Build history of the part. All positions in model axes, mm. Face numbers are marked on the shaded views. A direction names the side the tool comes from. Coordinates: 2 decimals unless noted, no trailing zeros. Loops run counter-clockwise (first coordinate to the right, second up) from the corner with the lowest first, then second, coordinate; pieces in that order, holes last.
Item 1: Mould opens along X. For the marked faces 4, 5 and 6 say: released by +X, released by -X, zero draft, split by the parting line, or undercut.
Item 2: Cut at D-D (x = 26). List the corners of the cut face in (y, z).
Item 3: Cut at A-A (x = 0). List the corners of the cut face in (y, z).
Item 4: Cut at B-B (z = -21). List the corners of the cut face in (x, y).
Item 5: 3-axis set-ups, long thin cutter, end or side, ignore diameter. For the marked faces 1, 2 and 3: which of +Z, -Z, +X, -X, +Y, -Y reach the whole face in a straight line?
Item 6: Flat gauge pins, fed straight in: pin 1 (3 mm diameter, centred on x = 30, y = -15, fed in from +Z); pin 2 (6.5 mm diameter, centred on x = 0, z = -21, fed in from +Y); pin 3 (24 mm diameter, centred on x = -20, y = -10.5, fed in from -Z); pin 4 (3 mm diameter, centred on x = 0, z = -21, fed in from -Y). Where does each tip first touch, or does it go through?
Item 7: Cut at C-C (y = 0). List the corners of the cut face in (x, z).
Item 8: Drill centre lines: line 1 along Z through (x, y) = (0, 3.05); line 2 along Y through (x, z) = (0, -24); line 3 along Z through (x, y) = (-27, 26). Where is each one in solid material? Low to high.
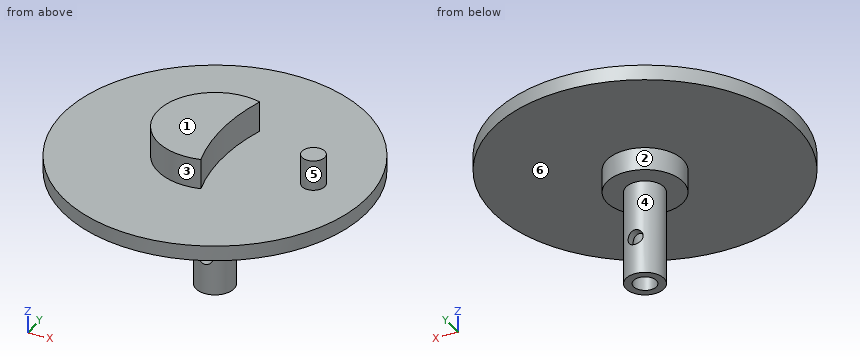
Autodesk Inventor part; units mm, degrees
ref_plane "YZ Plane" through (0, 0, 0) normal (1, 0, 0) x (0, 1, 0)
ref_plane "XZ Plane" through (0, 0, 0) normal (0, 1, 0) x (-1, 0, 0)
ref_plane "XY Plane" through (0, 0, 0) normal (0, 0, 1) x (1, 0, 0)
sketch "Sketch1" plane through (0, 0, 0) normal (0, 0, 1) x (1, 0, 0)
  circle A0 centre (0, 0) radius 40
  dimension "d0" = 40
extrude "Extrusion1" add sketch "Sketch1" along normal blind 4
sketch "Sketch2" plane through (0, 0, 4) normal (0, 0, 1) x (1, 0, 0)
  arc A0 (4.0325, 14.4478) -> (4.0325, -14.4478) centre (0, 0) ccw
  arc A1 (4.0325, 14.4478) -> (4.0325, -14.4478) centre (54.3652, 0) ccw
  dimension "d3" = 15
extrude "Extrusion2" add sketch "Sketch2" along normal blind 8
sketch "Sketch3" plane through (0, 0, 4) normal (0, 0, 1) x (1, 0, 0)
  circle A0 centre (26, 0) radius 3
  point P0 (0, 0)
  dimension "d6" = 3
sketch "Sketch4" plane through (0, 0, 0) normal (0, 0, -1) x (-1, 0, 0)
  circle A0 centre (0, 0) radius 10
  dimension "d9" = 10
extrude "Extrusion4" add sketch "Sketch4" along normal blind 6
sketch "Sketch5" plane through (0, 0, -6) normal (0, 0, -1) x (-1, 0, 0)
  circle A0 centre (0, 0) radius 5
  circle A1 centre (0, 0) radius 3
  dimension "d12" = 5
  dimension "d13" = 3
extrude "Extrusion5" add sketch "Sketch5" along normal blind 25
sketch "Sketch6" plane through (0, 0, 0) normal (0, 1, 0) x (-1, 0, 0)
  circle A0 centre (0, -21) radius 2
  point P0 (0, 0)
  dimension "d16" = 2
extrude "Extrusion6" cut sketch "Sketch6" along normal mid plane 25
extrude "Extrusion7" add sketch "Sketch3" along normal blind 8
properties part number "driverwheel"
Filled sheet:
1. face 4: split by the parting line
1. face 5: undercut
1. face 6: zero draft
2. outline: (-30.4, 0) - (30.4, 0) - (30.4, 4) - (3, 4) - (3, 12) - (-3, 12) - (-3, 4) - (-30.4, 4) - close
3. outline: (-40, 0) - (-10, 0) - (-10, -6) - (-5, -6) - (-5, -19) - (-3, -19) - (-3, -6) - (3, -6) - (3, -19) - (5, -19) - (5, -6) - (10, -6) - (10, 0) - (40, 0) - (40, 4) - (15, 4) - (15, 12) - (-15, 12) - (-15, 4) - (-40, 4) - close; (-5, -31) - (-3, -31) - (-3, -23) - (-5, -23) - close; (3, -31) - (5, -31) - (5, -23) - (3, -23) - close
4. outline: (-2, -4.58) - (-2, -2.24) arc R3 cw to (-2, 2.24) - (-2, 4.58) arc R5 ccw to start; (2, -4.58) arc R5 ccw to (2, 4.58) - (2, 2.24) arc R3 cw to (2, -2.24) - close
5. face 1: +Z, +X, -X, +Y, -Y
5. face 2: -Z
5. face 3: +Z
6. pin 1: stops at z = 4
6. pin 2: stops at y = 5
6. pin 3: stops at z = 0
6. pin 4: passes through
7. outline: (-40, 0) - (-10, 0) - (-10, -6) - (-5, -6) - (-5, -31) - (-3, -31) - (-3, -6) - (3, -6) - (3, -31) - (5, -31) - (5, -6) - (10, -6) - (10, 0) - (40, 0) - (40, 4) - (29, 4) - (29, 12) - (23, 12) - (23, 4) - (2, 4) - (2, 12) - (-15, 12) - (-15, 4) - (-40, 4) - close
8. line 1: z = -31 to -23, -19 to 12
8. line 2: y = -5 to -3, 3 to 5
8. line 3: z = 0 to 4
